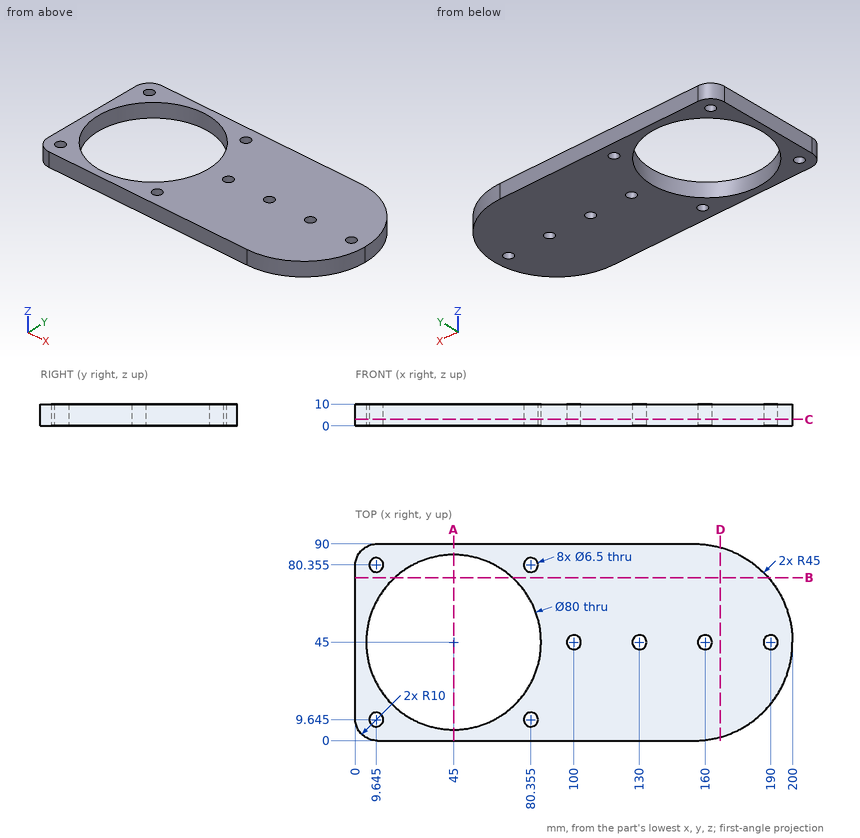
Verification items for this drawing (mm, ordinates from the low corner). Coordinates: 2 decimals unless noted, no trailing zeros. Loops run counter-clockwise (first coordinate to the right, second up) from the corner with the lowest first, then second, coordinate; pieces in that order, holes last.
Item 1: Sectioned sample at B-B, the plane y = 74.5. Record the boundary of the cut face in (x, z), then the cut area to 3 significant figures.
Item 2: Sectioned sample at D-D, the plane x = 167. Record the boundary of the cut face in (y, z).
Item 3: Sectioned sample at C-C, the plane z = 3. Count the separate pieces of the cut face and the enclosed holes in it, then the cut area to 3 significant figures.
Item 4: Thickness scan on line 1 (Y direction, x = 130, z = 5); line 2 (Y direction, x = 50, z = 5.75); line 3 (X direction, y = 21.5, z = 7) (1 decimal). Record the ranges inside material, lowest first.
Item 5: Go/stop test with flat-tipped pins: pin 1 Ø1 at (x, z) = (172.5, 7) entering from -Y (1 decimal); pin 2 Ø3 at (y, z) = (75, 4) entering from +X (1 decimal); pin 3 Ø6 at (y, z) = (22, 5) entering from +X. Record where each tip stops, or that it passes through.
Item 6: Sectioned sample at A-A, the plane x = 45. Record the boundary of the cut face in (y, z).
Check result:
1. outline: (0, 0) - (17.99, 0) - (17.99, 10) - (0, 10) - close; (72.01, 0) - (188.98, 0) - (188.98, 10) - (72.01, 10) - close
1. area: 1,350 mm2
2. outline: (1.63, 0) - (88.37, 0) - (88.37, 10) - (1.63, 10) - close
3. separate pieces: 1
3. enclosed holes: 9
3. area: 11,800 mm2
4. line 1: y = 0 to 41.75, 48.25 to 90
4. line 2: y = 0 to 5.31, 84.69 to 90
4. line 3: x = 0 to 12.6, 77.4 to 193.4
5. pin 1: stops at y = 3.3
5. pin 2: stops at x = 189.8
5. pin 3: stops at x = 195.31
6. outline: (0, 0) - (5, 0) - (5, 10) - (0, 10) - close; (85, 0) - (90, 0) - (90, 10) - (85, 10) - close
